from build123d import *

# Parameters (mm, degrees)
SKETCH1_R           = 2.1
SKETCH1_R_2         = 1.6
BOSS_EXTRUDE1_DEPTH = 3


with BuildPart() as part:
    # Sketch1 → Boss-Extrude1 (new body)
    with BuildSketch(Plane.XY):
        with BuildLine():
            Line((41, 136.6), (41, 125.6))
            ThreePointArc((41, 125.6), (41.878679656, 123.478679656), (44, 122.6))
            Line((44, 122.6), (47, 122.6))
            Line((47, 122.6), (47, -29.8))
            Line((47, -29.8), (10, -29.8))
            Line((10, -29.8), (10, -12.5))
            Line((10, -12.5), (0, -12.5))
            ThreePointArc((0, -12.5), (-12.5, 0), (0, 12.5))
            Line((0, 12.5), (16, 12.5))
            Line((16, 12.5), (16, 104.5))
            Line((16, 104.5), (0, 104.5))
            ThreePointArc((0, 104.5), (-8.838834765, 108.161165235), (-12.5, 117))
            Line((-12.5, 117), (-12.5, 124.1))
            ThreePointArc((-12.5, 124.1), (-8.838834765, 132.938834765), (0, 136.6))
            Line((0, 136.6), (41, 136.6))
        make_face()
        Circle(SKETCH1_R, mode=Mode.SUBTRACT)
        with Locations((0, 117)):
            Circle(SKETCH1_R, mode=Mode.SUBTRACT)
        with Locations((13.2, -21.3)):
            Circle(SKETCH1_R_2, mode=Mode.SUBTRACT)
        with Locations((24.5, 134)):
            Circle(SKETCH1_R_2, mode=Mode.SUBTRACT)
    extrude(amount=BOSS_EXTRUDE1_DEPTH)


solid = part.part
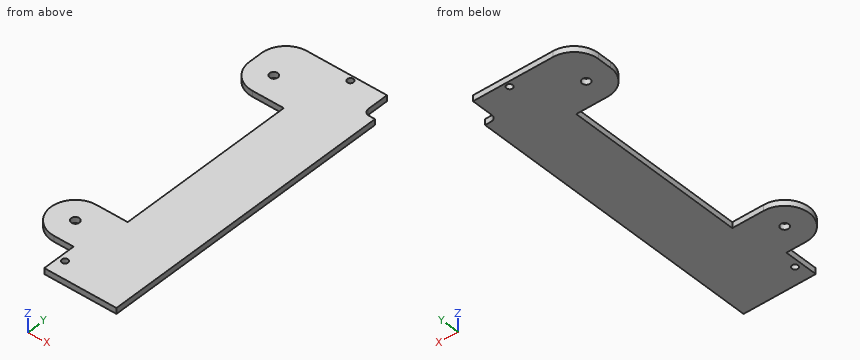
Part model, mm, in its own coordinate system. Coordinates: 2 decimals unless noted, no trailing zeros. Loops run counter-clockwise (first coordinate to the right, second up) from the corner with the lowest first, then second, coordinate; pieces in that order, holes last. Notation, with made-up numbers: (-13, -10.75) -> (4, -10.75) arc R19 ccw to (4, 1.25) -> close; hole circle Ø3 at (74, 23). An arc over 180 degrees is marked (long way). Use a Markdown table: item, result. Add a question column.
Item 1: Band-saw the part on B-B on y = 0. Write the cut outline in (x, z), plus the area to 3 significant figures.
Item 2: Flat gauge pins, fed straight in: P1, Ø1.5, axis at x = 9, z = 1.5, coming from the -Y side; P2, Ø0.9, axis at x = 45, z = 1, coming from the +Y side; P3, Ø1.9, axis at x = 24.5, y = 134, coming from the -Z side; P4, Ø0.9, axis at y = 51.5, z = 1, coming from the -X side. Where does each tip first touch, or does it go through?
Item 3: Band-saw the part on C-C on x = 24.5. Write the cut outline in (y, z), plus the area to 3 significant figures.
Item 4: Probe probe 1 along Y at (x, z) = (0, 2.4); probe 2 along X at (y, z) = (-17, 2.75); probe 3 along Y at (x, z) = (24.5, 1.75). List the from-to ranges inside material, lowest first.
Item 5: Band-saw the part on A-A on x = 13.2. Write the cut outline in (y, z), plus the area to 3 significant figures.
Item 6: Band-saw the part on D-D on z = 1. Write the cut outline in (x, y).
Geometry says:
| question | item | result |
|---|---|---|
| 1 | outline | (-12.5, 0) -> (-2.1, 0) -> (-2.1, 3) -> (-12.5, 3) -> close; (2.1, 0) -> (47, 0) -> (47, 3) -> (2.1, 3) -> close |
| 1 | area | 166 mm² |
| 2 | P1 | y = -12.5 |
| 2 | P2 | y = 122.6 |
| 2 | P3 | through |
| 2 | P4 | x = 16 |
| 3 | outline | (-29.8, 0) -> (132.4, 0) -> (132.4, 3) -> (-29.8, 3) -> close; (135.6, 0) -> (136.6, 0) -> (136.6, 3) -> (135.6, 3) -> close |
| 3 | area | 490 mm² |
| 4 | probe 1 | -12.5 to -2.1, 2.1 to 12.5, 104.5 to 114.9, 119.1 to 136.6 |
| 4 | probe 2 | 10 to 47 |
| 4 | probe 3 | -29.8 to 132.4, 135.6 to 136.6 |
| 5 | outline | (-29.8, 0) -> (-22.9, 0) -> (-22.9, 3) -> (-29.8, 3) -> close; (-19.7, 0) -> (12.5, 0) -> (12.5, 3) -> (-19.7, 3) -> close; (104.5, 0) -> (136.6, 0) -> (136.6, 3) -> (104.5, 3) -> close |
| 5 | area | 214 mm² |
| 6 | outline | (-12.5, 117) arc R12.5 ccw to (0, 104.5) -> (16, 104.5) -> (16, 12.5) -> (0, 12.5) arc R12.5 ccw to (0, -12.5) -> (10, -12.5) -> (10, -29.8) -> (47, -29.8) -> (47, 122.6) -> (44, 122.6) arc R3 cw to (41, 125.6) -> (41, 136.6) -> (0, 136.6) arc R12.5 ccw to (-12.5, 124.1) -> close; hole circle Ø4.2 at (0, 0); hole circle Ø4.2 at (0, 117); hole circle Ø3.2 at (13.2, -21.3); hole circle Ø3.2 at (24.5, 134) |
